from build123d import *

# Parameters (mm, degrees)
F0_W     = 38.1
F0_H     = 25.4
F1_DEPTH = 25.4
F2_W     = 12.7
F2_H     = 19.05
F3_DEPTH = 19.05
F4_ANGLE = 180


with BuildPart() as f1:
    # F0 (on Top) → F1 (new body)
    with BuildSketch(Plane.XY):
        with Locations((19.05, 12.7)):
            Rectangle(F0_W, F0_H)
    extrude(amount=F1_DEPTH)

    # F2 (on Right) → F3 (cut)
    with BuildSketch(Plane.YZ):
        with Locations((12.7, 16.149852)):
            Rectangle(F2_W, F2_H)
    extrude(amount=F3_DEPTH, mode=Mode.SUBTRACT)


with BuildPart() as f1_1:
    # F4: moved
    add(f1.part.rotate(Axis((38.1, 0, 12.7), (0, 0, 1)), F4_ANGLE))


solid = f1_1.part
Source: CAD feature listing. Evaluate the final solid. Frame: model axes, mm. A direction names the side the tool comes from. Round coordinates to 2 decimals unless told otherwise and drop trailing zeros. Loops run counter-clockwise (first coordinate to the right, second up) from the corner with the lowest first, then second, coordinate; pieces in that order, holes last. Notation, with made-up numbers: (-15.5, 17) - (24.5, 17) arc R21 cw to (24.5, 51) - close; hole circle Ø1 at (68, -0.5). An arc over 180 degrees is marked (long way). Write item = value, one per line. Start each with the question number.
Item 1: First-contact query: pin 1 Ø4 at (y, z) = (-11, 14.5) entering from +X. Flat tip, straight axial feed; report the tip coordinate or a pass-through.
Item 2: Section query A-A on x = 61. Output: boundary loops of the cut face in (y, z), plus the area to 3 significant figures.
Item 3: Reachability of faces 1 (the face through (57.15, -13, 16)), 2 (the face through (57, -13, 0)) from +Z, -Z, +X, -X, +Y, -Y: full face, straight path, thin tool, end or side. Return the list, or none.
Item 4: Mould query, pull axis Y, two halves, no side actions, for faces 3 (the face through (67, -19.05, 16)), 4 (the face through (57, 0, 13)), 5 (the face through (53, -13, 25.4)). Classes: released by +Y, released by -Y, zero draft, split by the parting line, or undercut.
Item 5: Material intervals for line 1 (Y direction, x = 67.5, z = 15.25); line 2 (X direction, y = -13, z = 14); line 3 (Z direction, x = 63.5, y = -13.5), sorted ascending.
Item 6: Section query B-B on y = -13.5. Output: boundary loops of the cut face in (x, z), plus the area to 3 significant figures.
Item 7: Section query C-C on z = 17. Output: boundary loops of the cut face in (x, y).
Results list:
q1.pin_1 = 57.15
q2.outline = (-25.4, 0) - (0, 0) - (0, 25.4) - (-6.35, 25.4) - (-6.35, 6.62) - (-19.05, 6.62) - (-19.05, 25.4) - (-25.4, 25.4) - close
q2.area = 407 mm²
q3.face_1 = +Z, +X
q3.face_2 = -Z, +X, -X, +Y, -Y
q4.face_3 = undercut
q4.face_4 = released by +Y
q4.face_5 = zero draft
q5.line_1 = -25.4 to -19.05, -6.35 to 0
q5.line_2 = 38.1 to 57.15
q5.line_3 = 0 to 6.62
q6.outline = (38.1, 0) - (76.2, 0) - (76.2, 6.62) - (57.15, 6.62) - (57.15, 25.4) - (38.1, 25.4) - close
q6.area = 610 mm²
q7.outline = (38.1, -25.4) - (76.2, -25.4) - (76.2, -19.05) - (57.15, -19.05) - (57.15, -6.35) - (76.2, -6.35) - (76.2, 0) - (38.1, 0) - close
